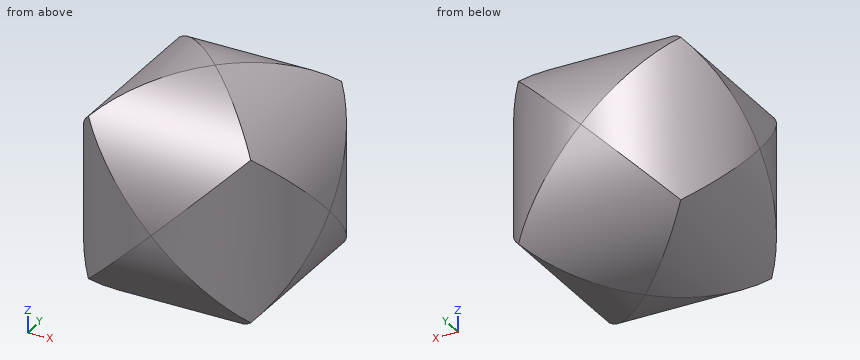
from build123d import *

# Parameters (mm, degrees)
F0_R     = 7.5
F3_DEPTH = 7.5
F1_R     = 7.5
F4_DEPTH = 7.5
F2_R     = 7.5
F5_DEPTH = 7.5


with BuildPart() as f3:
    # F0 (on Front) → F3 (new body, symmetric)
    with BuildSketch(Plane.XZ):
        Circle(F0_R)
    extrude(amount=F3_DEPTH, both=True)

    # F1 (on Top) → F4 (intersect, symmetric)
    with BuildSketch(Plane.XY):
        Circle(F1_R)
    extrude(amount=F4_DEPTH, both=True, mode=Mode.INTERSECT)

    # F2 (on Right) → F5 (intersect, symmetric)
    with BuildSketch(Plane.YZ):
        Circle(F2_R)
    extrude(amount=F5_DEPTH, both=True, mode=Mode.INTERSECT)


solid = f3.part
CAD build for the part. Positions are in the model's coordinates, mm. Coordinates: 2 decimals unless noted, no trailing zeros. Write each loop counter-clockwise with the first axis right and the second up, starting at its lowest first coordinate (ties: lowest second). Pieces come first, ordered by that corner, then holes. Notation, with made-up numbers: M -11.5,-38.5 L -6.5,-38.5 A20 cw -6.5,-2.5 Z; hole C -6,68.5 d6. An arc over 180 degrees is marked long. Return JSON: item names as keys, results as strings.
Item 1: Slice it at C-C, the plane y = 6. Write the cut outline in (x, z).
Findings below:
{"outline": "M -4.5,-4.5 L 4.5,-4.5 L 4.5,4.5 L -4.5,4.5 Z"}
Item 2: Slice it at A-A, the plane y = 4.5. Write the cut outline in (x, z).
Findings below:
{"outline": "M -6,-4.5 A7.5 ccw -4.5,-6 L 4.5,-6 A7.5 ccw 6,-4.5 L 6,4.5 A7.5 ccw 4.5,6 L -4.5,6 A7.5 ccw -6,4.5 Z"}
Item 3: Drop flat-ended pins along their axis: pin 1 Ø8 at (x, z) = (0, 6) entering from -Y; pin 2 Ø1 at (x, z) = (1.5, 4.5) entering from -Y; pin 3 Ø3 at (y, z) = (-1, 6) entering from -X. Give the stop position or say it passes through.
Findings below:
{"pin 1": "stops at y = -7.23", "pin 2": "stops at y = -6.34", "pin 3": "stops at x = -6"}
Item 4: Slice it at D-D, the plane x = 6.75. Write the cut outline in (y, z).
Findings below:
{"outline": "M -3.27,-3.27 L 3.27,-3.27 L 3.27,3.27 L -3.27,3.27 Z"}
Item 5: Probe line 1 (X direction, y = -1, z = 6.25); line 2 (Y direction, x = -6, z = -0.25); line 3 (Z direction, x = 0, y = -1). List the from-to ranges inside material, lowest first. Write a range as from..to.
Findings below:
{"line 1": "x = -4.15..4.15", "line 2": "y = -4.5..4.5", "line 3": "z = -7.43..7.43"}
Item 6: Slice it at B-B, the plane x = 2. Write the cut outline in (y, z), and give its area (3 significant figures).
Findings below:
{"outline": "M -7.23,-2 A7.5 ccw -2,-7.23 L 2,-7.23 A7.5 ccw 7.23,-2 L 7.23,2 A7.5 ccw 2,7.23 L -2,7.23 A7.5 ccw -7.23,2 Z", "area": "174 mm2"}
